Geometry: final body of the model. Coordinates: model frame, mm. Give positions to 0.01 mm unless a question says otherwise; leave off trailing zeros. Loops run counter-clockwise (first coordinate to the right, second up) from the corner with the lowest first, then second, coordinate; pieces in that order, holes last.
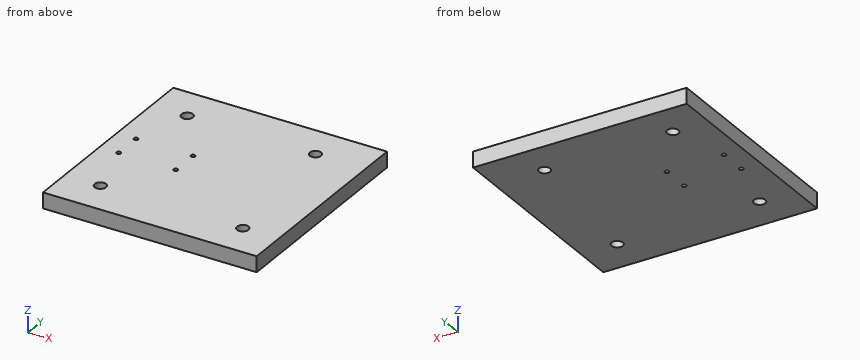
Autodesk Inventor part; units mm, degrees
ref_plane "YZ Plane" through (0, 0, 0) normal (1, 0, 0) x (0, 1, 0)
ref_plane "XZ Plane" through (0, 0, 0) normal (0, 1, 0) x (-1, 0, 0)
ref_plane "XY Plane" through (0, 0, 0) normal (0, 0, 1) x (1, 0, 0)
sketch "Sketch1" plane through (0, 0, 0) normal (0, 0, 1) x (1, 0, 0)
  line L0 (0, 0) -> (150, 0)
  line L1 (150, 0) -> (150, 150)
  line L2 (150, 150) -> (0, 150)
  line L3 (0, 150) -> (0, 0)
  dimension "d0" = 150
  dimension "d1" = 150
extrude "Extrusion1" add sketch "Sketch1" along normal blind 11
sketch "Sketch2" plane through (0, 0, 11) normal (0, 0, 1) x (1, 0, 0)
  circle A0 centre (13.5, 85) radius 1.5
  circle A1 centre (13.5, 65) radius 1.5
  circle A2 centre (53.5, 85) radius 1.5
  circle A3 centre (53.5, 65) radius 1.5
  line L0 (0, 150) -> (0, 0)
  line L1 (0, 0) -> (150, 0)
  line L2 (150, 150) -> (0, 150)
  line L3 (75, 150) -> (75, 0)
  line L4 (-23.1394, 75) -> (177.6706, 75)
  dimension "d4" = 3
  dimension "d5" = 3
  dimension "d6" = 20
  dimension "d7" = 3
  dimension "d8" = 3
  dimension "d10" = 40
  dimension "d11" = 40
  dimension "d12" = 20
  dimension "d13" = 13.5
  dimension "d14" = 13.5
  dimension "d15" = 65
  dimension "d16" = 65
extrude "Extrusion2" cut sketch "Sketch2" against normal blind 11 contours A0 | A1 | A2 | A3
sketch "Sketch3" plane through (0, 0, 11) normal (0, 0, 1) x (1, 0, 0)
  circle A0 centre (25, 25) radius 4
  circle A1 centre (25, 125) radius 4
  circle A2 centre (125, 25) radius 4
  circle A3 centre (115, 125) radius 4
  line L0 (150, 0) -> (150, 150)
  line L1 (150, 150) -> (0, 150)
  line L2 (0, 0) -> (150, 0)
  line L3 (0, 150) -> (0, 0)
  dimension "d19" = 8
  dimension "d20" = 8
  dimension "d21" = 8
  dimension "d22" = 8
  dimension "d23" = 35
  dimension "d24" = 25
  dimension "d25" = 25
  dimension "d26" = 25
  dimension "d27" = 25
  dimension "d28" = 25
  dimension "d29" = 25
  dimension "d30" = 25
extrude "Extrusion3" cut sketch "Sketch3" against normal blind 11 contours A0 | A1 | A2 | A3
properties part number "Teste bloco do motor"
Item 1: Ray query, probe 1 along Y at (x, z) = (13.5, 8.25); probe 2 along X at (y, z) = (65, 7.5); probe 3 along Y at (x, z) = (25, 4.5). Return the intervals inside material, ascending.
Values follow:
probe 1: y = 0 to 63.5, 66.5 to 83.5, 86.5 to 150
probe 2: x = 0 to 12, 15 to 52, 55 to 150
probe 3: y = 0 to 21, 29 to 121, 129 to 150
Item 2: Section query A-A on x = 25. Return loops of the section in (y, z), plus the area to 3 significant figures.
Values follow:
outline: (0, 0) - (21, 0) - (21, 11) - (0, 11) - close; (29, 0) - (121, 0) - (121, 11) - (29, 11) - close; (129, 0) - (150, 0) - (150, 11) - (129, 11) - close
area: 1,470 mm2
